Autodesk Inventor part; units mm, degrees
ref_plane "YZ Plane" through (0, 0, 0) normal (1, 0, 0) x (0, 1, 0)
ref_plane "XZ Plane" through (0, 0, 0) normal (0, 1, 0) x (-1, 0, 0)
ref_plane "XY Plane" through (0, 0, 0) normal (0, 0, 1) x (1, 0, 0)
sketch "Sketch1" plane through (0, 0, 0) normal (0, 0, 1) x (1, 0, 0)
  line L0 (-16.5, 11) -> (16.5, 11)
  line L1 (16.5, 11) -> (16.5, -11)
  line L2 (16.5, -11) -> (-16.5, -11) construction
  line L3 (-16.5, -11) -> (-16.5, 11)
  line L4 (-16.5, 11) -> (16.5, -11) construction
  line L5 (16.5, 11) -> (-16.5, -11) construction
  line L6 (-16.5, -11) -> (-1.5, -11)
  line L7 (-1.5, -11) -> (-1.5, -33)
  line L8 (-1.5, -33) -> (16.5, -33)
  line L9 (16.5, -33) -> (16.5, -11)
  circle A0 centre (0, 0) radius 5.15
  circle A1 centre (0, 8) radius 1.05
  circle A2 centre (-8, 0) radius 1.05
  circle A3 centre (0, -8) radius 1.05
  circle A4 centre (8, 0) radius 1.05
  dimension "d0" = 33
  dimension "d1" = 22
  dimension "d2" = 15
  dimension "d3" = 44
  dimension "d4" = 10.3
  dimension "d5" = 8
  dimension "d8" = 360
  dimension "d10" = 2.1
extrude "Extrusion1" add sketch "Sketch1" along normal blind 9
sketch "Sketch2" plane through (-16.5, -11, 0) normal (-1, 0, 0) x (0, 0, 1)
  circle A0 centre (4.5, 4) radius 1.5
  line L0 (0, 0) -> (9, 0) construction
  line L1 (9, 22) -> (9, 0)
  line L2 (0, 11) -> (9, 11) construction
  line L3 (0, 22) -> (0, 0)
  circle A1 centre (4.5, 18) radius 1.5
  point P0 (0, 11)
  point P1 (4.5, 0)
  dimension "d13" = 3
  dimension "d14" = 4
extrude "Extrusion2" cut sketch "Sketch2" against normal blind 5
properties part number "batente_microswitch_001" material "ABS Plastic"
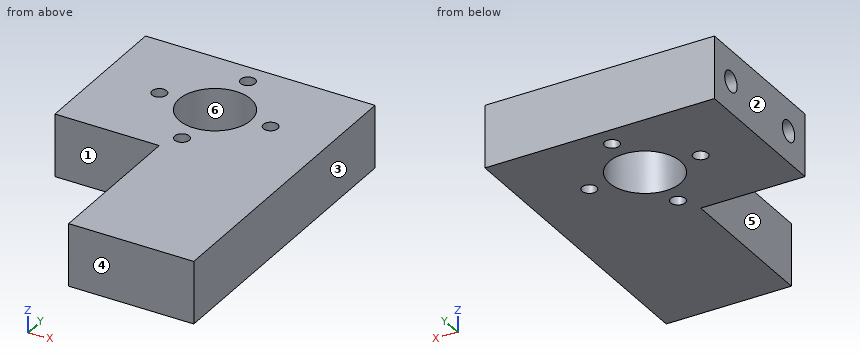
The listing builds one solid part. Answer for the finished solid, in the listing's coordinates (mm). Face numbers are marked on the shaded views. A direction names the side the tool comes from. Round coordinates to 2 decimals unless told otherwise and drop trailing zeros. Write each loop counter-clockwise with the first axis right and the second up, starting at its lowest first coordinate (ties: lowest second). Pieces come first, ordered by that corner, then holes. Notation, with made-up numbers: (-2.5, -18) -> (27.5, -18) arc R13 cw to (27.5, -11) -> close; hole circle Ø8 at (26.5, 9). An arc over 180 degrees is marked (long way). Write item = value, one per line.
1) Which of the six approach directions +Z, -Z, +X, -X, +Y, -Y give full straight-line access (tool end or side, diameter ignored) to the marked faces 1 and 2?
Check values:
face_1 = +Z, -Z, -X, -Y
face_2 = +Z, -Z, -X, +Y, -Y
2) For a pull along X with two mould halves and no side action, classify the marked faces 3, 4, 5 and 6 as released by +X, released by -X, zero draft, split by the parting line, or undercut.
Check values:
face_3 = released by +X
face_4 = zero draft
face_5 = released by -X
face_6 = undercut
3) Section D-D on x = 8 is taken. Write down the section's boundary in (y, z).
Check values:
outline = (-33, 0) -> (-1.05, 0) -> (-1.05, 9) -> (-33, 9) -> close; (1.05, 0) -> (11, 0) -> (11, 9) -> (1.05, 9) -> close
4) Section B-B on z = 1.5 is taken. Write down the section's boundary in (x, y).
Check values:
outline = (-16.5, -11) -> (-1.5, -11) -> (-1.5, -33) -> (16.5, -33) -> (16.5, 11) -> (-16.5, 11) -> close; hole circle Ø2.1 at (-8, 0); hole circle Ø10.3 at (0, 0); hole circle Ø2.1 at (0, -8); hole circle Ø2.1 at (0, 8); hole circle Ø2.1 at (8, 0)
5) Section C-C on y = 3 is taken. Write down the section's boundary in (x, z).
Check values:
outline = (-16.5, 0) -> (-4.19, 0) -> (-4.19, 9) -> (-16.5, 9) -> close; (4.19, 0) -> (16.5, 0) -> (16.5, 9) -> (4.19, 9) -> close
6) Section A-A on x = 0 is taken. Write down the section's boundary in (y, z), plus the area to 4 significant figures.
Check values:
outline = (-33, 0) -> (-9.05, 0) -> (-9.05, 9) -> (-33, 9) -> close; (-6.95, 0) -> (-5.15, 0) -> (-5.15, 9) -> (-6.95, 9) -> close; (5.15, 0) -> (6.95, 0) -> (6.95, 9) -> (5.15, 9) -> close; (9.05, 0) -> (11, 0) -> (11, 9) -> (9.05, 9) -> close
area = 265.5 mm²
7) Given pin 1 (1.5 mm diameter, centred on y = -7.5, z = 5, fed in from -X); pin 2 (4.5 mm diameter, centred on y = -17.5, z = 3.5, fed in from -X); pin 3 (1.5 mm diameter, centred on x = -6.5, z = 6.5, fed in from -Y), each flat-ended and moving along its own axis, determine where each tip first touches the part or whether it passes through.
Check values:
pin_1 = -11.5
pin_2 = -1.5
pin_3 = -11
8) Straight lines are drawn through the part: line 1 along Y through (x, z) = (0, 2); line 2 along Y through (x, z) = (-13.25, 4.5); line 3 along Y through (x, z) = (-8, 4.5). For each, find the intervals that lie inside material, in ascending order. Write a range as [from, to].
Check values:
line_1 = [-33, -9.05], [-6.95, -5.15], [5.15, 6.95], [9.05, 11]
line_2 = [-11, -8.5], [-5.5, 5.5], [8.5, 11]
line_3 = [-11, -1.05], [1.05, 11]
